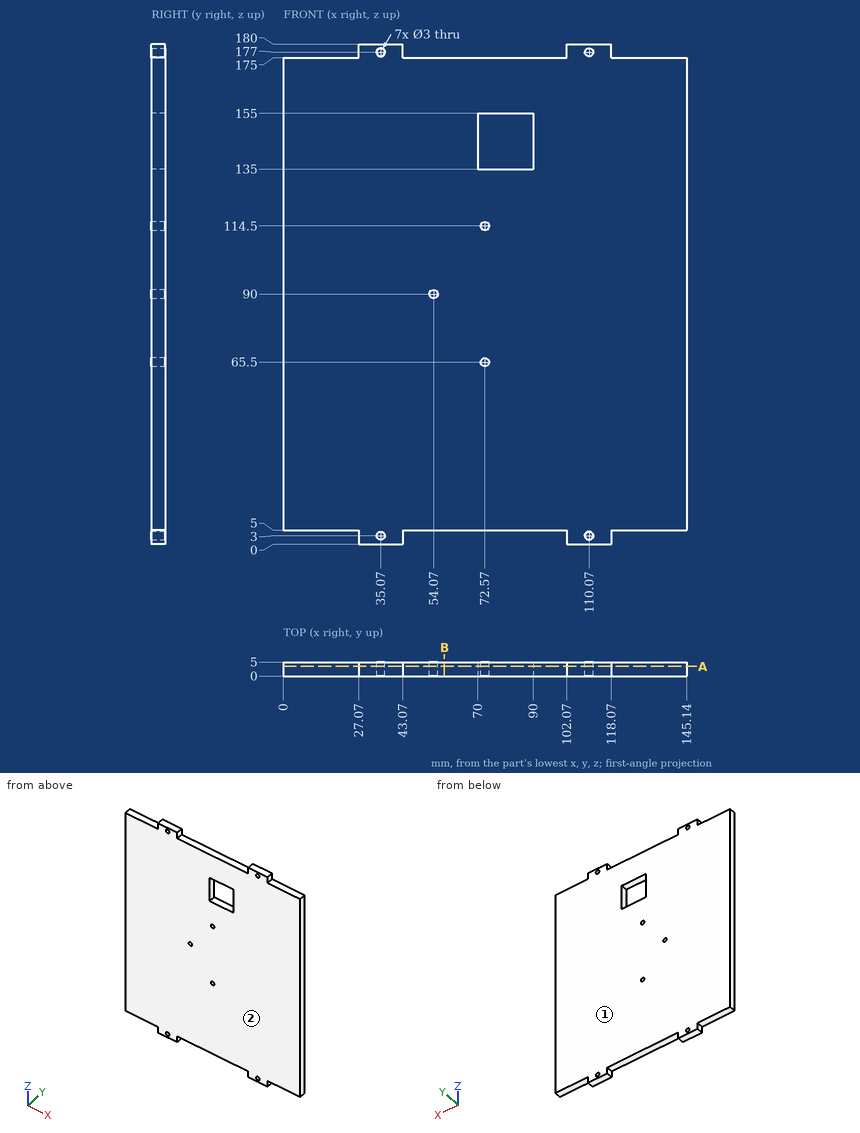
Design review of the part shown in the three views and the two pictorial views. Dimensions are in mm from the part's minimum x, y and z. Give positions to 0.01 mm unless a question says otherwise; leave off trailing zeros. Write each loop counter-clockwise with the first axis right and the second up, starting at its lowest first coordinate (ties: lowest second). Pieces come first, ordered by that corner, then holes. Notation, with made-up numbers: M 42.25,2.25 L 57.25,2.25 A29 cw 57.25,38.25 Z; hole C 49,84.5 d6. An arc over 180 degrees is marked long. One line per question, with ' | ' between items. Start each with the question number.
Item 1: For pin 1 (1.5 mm diameter, centred on y = 2.5, z = 3.5, fed in from -X); pin 2 (2.5 mm diameter, centred on x = 11, y = 3.5, fed in from -Z), all flat-tipped, find the tip position at first contact; note any pin that passes through.
Item 2: Draft analysis for pull direction Y (two halves, no side actions). For the marked faces 1 and 2, state which applies: released by +Y, released by -Y, zero draft, split by the parting line, or undercut.
Item 3: We need section A-A on y = 3.45. Give the number of separate pieces and of enclosed holes in the cut face, plus the area to 3 significant figures.
Item 4: We need section B-B on x = 58. Write out the cut boundary in (y, z).
Item 5: Wall thickness on line 1 (X direction, y = 3.2, z = 177); line 2 (Z direction, x = 72.57, y = 2.1); line 3 (Z direction, x = 110.07, y = 2.15): over which ranges is each line inside the solid? List them lowest first. Write a range as from..to.
Results found:
1) pin 1: stops at x = 27.07 | pin 2: stops at z = 5
2) face 1: released by +Y | face 2: released by -Y
3) separate pieces: 1 | enclosed holes: 8 | area: 24,500 mm2
4) outline: M 0,5 L 5,5 L 5,175 L 0,175 Z
5) line 1: x = 27.07..33.57, 36.57..43.07, 102.07..108.57, 111.57..118.07 | line 2: z = 5..64, 67..113, 116..135, 155..175 | line 3: z = 0..1.5, 4.5..175.5, 178.5..180
